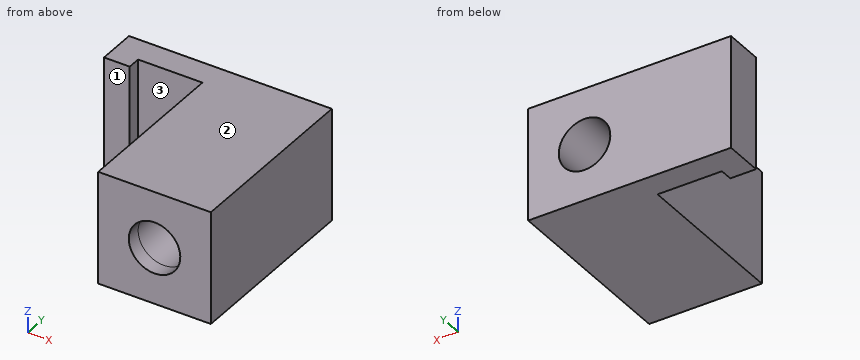
Solid Edge part; units mm, degrees
sketch "Sketch1" plane through (0, 0, 0) normal (0, 0, 1) x (1, 0, 0)
  line L0 (0, 10) -> (0, 9.2)
  line L1 (-1.6, 9.2) -> (0, 9.2)
  line L2 (-1.6, 11.6) -> (-1.6, 9.2)
  line L3 (10.1, 11.6) -> (-1.6, 11.6)
  line L4 (10.1, 0.9) -> (10.1, 11.6)
  line L5 (10.1, 0) -> (10.1, 0.9)
  line L6 (7.5, 0) -> (10.1, 0)
  line L7 (4, 0) -> (7.5, 0)
  line L8 (4, 10) -> (4, 0)
  line L9 (0, 10) -> (4, 10)
extrude "Protrusion1" add sketch "Sketch1" along normal blind 7
hole "Hole_1" at (7.5, 0.9, 3.5) direction (0, -1, 0) diameter 3.2 end up to next
sketch "Sketch2" plane through (7.5, 0.9, 3.5) normal (0, -1, 0) x (0, 0, -1)
  circle A0 centre (0, 0) radius 1.6
extrude "Cutout1" cut sketch "Sketch2" against normal up to next
sketch "Sketch3" plane through (10.1, 5.8, 3.5) normal (1, 0, 0) x (0, 1, 0)
  line L0 (-5.8, 3.5) -> (5.8, 3.5)
  line L1 (5.8, 3.5) -> (5.8, -3.5)
  line L2 (5.8, -3.5) -> (-5.8, -3.5)
  line L3 (-5.8, -3.5) -> (-5.8, 3.5)
extrude "ExtrudedProtrusion_2" add sketch "Sketch3" along normal blind 0.9
Verification items for the finished model (mm, model axes). Face numbers are marked on the shaded views. A direction names the side the tool comes from. Coordinates: 2 decimals unless noted, no trailing zeros. Loops run counter-clockwise (first coordinate to the right, second up) from the corner with the lowest first, then second, coordinate; pieces in that order, holes last. Notation, with made-up numbers: (-31, -28.5) - (-6, -28.5) arc R29 ccw to (-6, 3.5) - close; hole circle Ø3 at (76.5, 21). An arc over 180 degrees is marked (long way). Return JSON: item names as keys, results as strings.
1. Section check A-A, the plane z = 3.5. Record the boundary of the cut face in (x, y).
Established:
{"outline": "(-1.6, 9.2) - (0, 9.2) - (0, 10) - (4, 10) - (4, 0) - (5.9, 0) - (5.9, 11.6) - (-1.6, 11.6) - close; (9.1, 0) - (11, 0) - (11, 11.6) - (9.1, 11.6) - close"}
2. Tool access check on the marked faces 1, 2 and 3. Record the directions out of +Z, -Z, +X, -X, +Y, -Y that give a thin tool (end or side, any length) a straight path to the whole face; none if there is none.
Established:
{"face 1": "+Z, -Z, -X, -Y", "face 2": "+Z, +X, -X, +Y, -Y", "face 3": "+Z, -Z, -Y"}
3. Section check C-C, the plane y = 5.5. Record the boundary of the cut face in (x, z).
Established:
{"outline": "(4, 0) - (11, 0) - (11, 7) - (4, 7) - close; hole circle Ø3.2 at (7.5, 3.5)"}
4. Section check D-D, the plane z = 6.75. Record the boundary of the cut face in (x, y), then the cut area to 3 significant figures.
Established:
{"outline": "(-1.6, 9.2) - (0, 9.2) - (0, 10) - (4, 10) - (4, 0) - (11, 0) - (11, 11.6) - (-1.6, 11.6) - close", "area": "91.4 mm2"}
5. Thickness scan on L1, parallel to Z at x = 7.5, y = 7.75; L2, parallel to X at y = 4.25, z = 3.5; L3, parallel to Y at x = -0.25, z = 2. Record the ranges inside material, lowest first.
Established:
{"L1": "z = 0 to 1.9, 5.1 to 7", "L2": "x = 4 to 5.9, 9.1 to 11", "L3": "y = 9.2 to 11.6"}
6. Go/stop test with flat-tipped pins: pin 1 (1.9 mm diameter, centred on x = 7.5, z = 3.5, fed in from -Y); pin 2 (3 mm diameter, centred on x = 2, z = 2, fed in from -Y); pin 3 (1.3 mm diameter, centred on x = -1, z = 3.5, fed in from -Y). Record where each tip stops, or that it passes through.
Established:
{"pin 1": "passes through", "pin 2": "stops at y = 10", "pin 3": "stops at y = 9.2"}
7. Section check B-B, the plane x = 7.5. Record the boundary of the cut face in (y, z), then the cut area to 3 significant figures.
Established:
{"outline": "(0, 0) - (11.6, 0) - (11.6, 1.9) - (0, 1.9) - close; (0, 5.1) - (11.6, 5.1) - (11.6, 7) - (0, 7) - close", "area": "44.1 mm2"}
